from build123d import *

# Parameters (mm, degrees)
SKETCH_1_W          = 250
SKETCH_1_H          = 200
EXTRUDE_1_DEPTH     = 3.6
SKETCH_2_W          = 4
SKETCH_2_H          = 60
CUT_EXTRUDE_1_DEPTH = 10
SKETCH_3_W          = 60
SKETCH_3_H          = 4
CUT_EXTRUDE_2_DEPTH = 10
SKETCH_4_R          = 5
CUT_EXTRUDE_3_DEPTH = 10
SKETCH_5_W          = 250
SKETCH_5_H          = 3.6
EXTRUDE_2_DEPTH     = 4
SKETCH_6_W          = 60
SKETCH_6_H          = 4
CUT_EXTRUDE_4_DEPTH = 161.128073741
SKETCH_7_W          = 4
SKETCH_7_H          = 3.6
EXTRUDE_3_DEPTH     = 8.5
SKETCH_8_W          = 68.538276959
SKETCH_8_H          = 3.6
CUT_EXTRUDE_5_DEPTH = 8.5
SKETCH_9_W          = 8.538276959
SKETCH_9_H          = 4
EXTRUDE_4_DEPTH     = 4
SKETCH_10_W         = 60
SKETCH_10_H         = 4
CUT_EXTRUDE_6_DEPTH = 8.5


with BuildPart() as part:
    # 草图1 → 凸台-拉伸1 (new body)
    with BuildSketch(Plane.XY):
        Rectangle(SKETCH_1_W, SKETCH_1_H)
    extrude(amount=EXTRUDE_1_DEPTH)

    # 草图2 → 切除-拉伸1 (cut)
    with BuildSketch(Plane.XY.offset(3.6)):
        with Locations((-123, 55)):
            Rectangle(SKETCH_2_W, SKETCH_2_H)
        with Locations((123, 55)):
            Rectangle(SKETCH_2_W, SKETCH_2_H)
        with Locations((-123, -55)):
            Rectangle(SKETCH_2_W, SKETCH_2_H)
        with Locations((123, -55)):
            Rectangle(SKETCH_2_W, SKETCH_2_H)
    extrude(amount=-CUT_EXTRUDE_1_DEPTH, mode=Mode.SUBTRACT)

    # 草图3 → 切除-拉伸2 (cut)
    with BuildSketch(Plane.XY.offset(3.6)):
        with Locations((-55, -98)):
            Rectangle(SKETCH_3_W, SKETCH_3_H)
        with Locations((55, -98)):
            Rectangle(SKETCH_3_W, SKETCH_3_H)
        with Locations((55, 98)):
            Rectangle(SKETCH_3_W, SKETCH_3_H)
        with Locations((-55, 98)):
            Rectangle(SKETCH_3_W, SKETCH_3_H)
    extrude(amount=-CUT_EXTRUDE_2_DEPTH, mode=Mode.SUBTRACT)

    # 草图4 → 切除-拉伸3 (cut)
    with BuildSketch(Plane(origin=(0, 0, 0), x_dir=(-1, 0, 0), z_dir=(0, 0, -1))):
        with Locations((-63.5, 69.4)):
            Circle(SKETCH_4_R)
        with Locations((63.5, 69.4)):
            Circle(SKETCH_4_R)
    extrude(amount=-CUT_EXTRUDE_3_DEPTH, mode=Mode.SUBTRACT)

    # 草图5 → 凸台-拉伸2 (add)
    with BuildSketch(Plane(origin=(0, 0, 0), x_dir=(-1, 0, 0), z_dir=(0, 0, -1))):
        with Locations((0, 98.2)):
            Rectangle(SKETCH_5_W, SKETCH_5_H)
    extrude(amount=-EXTRUDE_2_DEPTH)

    # 草图6 → 切除-拉伸4 (cut, through all)
    with BuildSketch(Plane(origin=(0, 0, 0), x_dir=(-1, 0, 0), z_dir=(0, 0, -1))):
        with Locations((-55, 98)):
            Rectangle(SKETCH_6_W, SKETCH_6_H)
        with Locations((55, 98)):
            Rectangle(SKETCH_6_W, SKETCH_6_H)
    extrude(amount=-CUT_EXTRUDE_4_DEPTH, mode=Mode.SUBTRACT)

    # 草图7 → 凸台-拉伸3 (add)
    with BuildSketch(Plane(origin=(-85, 0, 0), x_dir=(0, 0, -1), z_dir=(1, 0, 0))):
        with Locations((-2, 98.2)):
            Rectangle(SKETCH_7_W, SKETCH_7_H)
    extrude(amount=EXTRUDE_3_DEPTH)

    # 草图8 → 切除-拉伸5 (cut)
    with BuildSketch(Plane(origin=(0, 0, 0), x_dir=(-1, 0, 0), z_dir=(0, 0, -1))):
        with Locations((50.717618655, 98.2)):
            Rectangle(SKETCH_8_W, SKETCH_8_H)
    extrude(amount=-CUT_EXTRUDE_5_DEPTH, mode=Mode.SUBTRACT)

    # 草图9 → 凸台-拉伸4 (add)
    with BuildSketch(Plane(origin=(0, 0, 0), x_dir=(-1, 0, 0), z_dir=(0, 0, -1))):
        with Locations((80.717618655, 98)):
            Rectangle(SKETCH_9_W, SKETCH_9_H)
    extrude(amount=-EXTRUDE_4_DEPTH)

    # 草图10 → 切除-拉伸6 (cut)
    with BuildSketch(Plane(origin=(0, 0, 0), x_dir=(-1, 0, 0), z_dir=(0, 0, -1))):
        with Locations((46.448480175, 98)):
            Rectangle(SKETCH_10_W, SKETCH_10_H)
    extrude(amount=-CUT_EXTRUDE_6_DEPTH, mode=Mode.SUBTRACT)


solid = part.part
Source: CAD feature listing. Evaluate the final solid. Frame: model axes, mm. Round coordinates to 2 decimals unless told otherwise and drop trailing zeros. Loops run counter-clockwise (first coordinate to the right, second up) from the corner with the lowest first, then second, coordinate; pieces in that order, holes last. Notation, with made-up numbers: (-33, -29) - (-20, -29) arc R28 cw to (-20, -9) - close; hole circle Ø10 at (37.25, -14). An arc over 180 degrees is marked (long way). Write item = value, one per line. Start each with the question number.
(1) Pull-direction query (X, two-part tool) for faces 1 (the face through (-62.849, 74.357, 1.775)), 2 (the face through (2, 1, 0)); classes: +X half, -X half, draft (parallel to the pull), parting line (faces both ways), or undercut.
(2) Pin query (flat end, axial travel): pin 1 (1.5 mm diameter, centred on x = -19.5, y = -3.5, fed in from +Z); pin 2 (1.8 mm diameter, centred on y = 41.5, z = 1.5, fed in from +X). Return the tip coordinate at first contact, or that it passes through.
(3) Section query B-B, the plane y = 69.4. Output: boundary loops of the cut face in (x, z), plus the area to 3 significant figures.
(4) Section query A-A, the plane x = -63.5. Output: boundary loops of the cut face in (y, z).
(5) Ray query, line 1 along Y through (x, z) = (-63.5, 2.55); line 2 along Z through (x, y) = (-90, -5.5); line 3 along Y through (x, z) = (-10.5, 3.7). Return the intervals inside material, ascending. Write a range as from..to.
(6) Section query D-D, the plane x = 90. Output: boundary loops of the cut face in (y, z), plus the area to 3 significant figures.
Conclusion:
q1.face_1 = undercut
q1.face_2 = draft
q2.pin_1 = 3.6
q2.pin_2 = 121
q3.outline = (-121, 0) - (-68.5, 0) - (-68.5, 3.6) - (-121, 3.6) - close; (-58.5, 0) - (58.5, 0) - (58.5, 3.6) - (-58.5, 3.6) - close; (68.5, 0) - (121, 0) - (121, 3.6) - (68.5, 3.6) - close
q3.area = 799 mm2
q4.outline = (-96, 0) - (64.4, 0) - (64.4, 3.6) - (-96, 3.6) - close; (74.4, 0) - (96, 0) - (96, 3.6) - (74.4, 3.6) - close
q5.line_1 = -96..64.4, 74.4..96
q5.line_2 = 0..3.6
q5.line_3 = 96.4..100
q6.outline = (-100, 0) - (100, 0) - (100, 4) - (96.4, 4) - (96.4, 3.6) - (-100, 3.6) - close
q6.area = 721 mm2
